Autodesk Inventor part; units mm, degrees
ref_plane "YZ Plane" through (0, 0, 0) normal (1, 0, 0) x (0, 1, 0)
ref_plane "XZ Plane" through (0, 0, 0) normal (0, 1, 0) x (-1, 0, 0)
ref_plane "XY Plane" through (0, 0, 0) normal (0, 0, 1) x (1, 0, 0)
sketch "Sketch1" plane through (0, 0, 0) normal (0, 1, 0) x (-1, 0, 0)
  line L0 (33.5, -13.5) -> (-33.5, -13.5)
  line L1 (-33.5, -13.5) -> (-33.5, 13.5)
  line L2 (-33.5, 13.5) -> (33.5, 13.5)
  line L3 (33.5, 13.5) -> (33.5, -13.5)
  line L4 (0, 0) -> (86.7229, 0) construction
  line L5 (0, 0) -> (0, 45.1017) construction
  dimension "d0" = 27
  dimension "d1" = 67
extrude "Extrusion1" add sketch "Sketch1" along normal blind 3
sketch "Sketch2" plane through (0, 3, 0) normal (0, 1, 0) x (1, 0, 0)
  line L0 (33.5, 13.5) -> (-33.5, 13.5)
  line L1 (33.5, -13.5) -> (33.5, 13.5)
  line L2 (0, 0) -> (26.8835, 0) construction
  line L3 (0, 0) -> (0, 11.9949) construction
  circle A0 centre (30, 9) radius 2.15
  circle A1 centre (-30, 9) radius 2.15
  circle A2 centre (30, -9) radius 2.15
  circle A3 centre (-30, -9) radius 2.15
  dimension "d4" = 4.3
  dimension "d5" = 3.5
  dimension "d6" = 4.5
extrude "Extrusion2" cut sketch "Sketch2" against normal through all
fillet "Fillet1" radius 2 4 edges at (-33.5, 1.5, 13.5) (-33.5, 1.5, -13.5) (33.5, 1.5, -13.5) (33.5, 1.5, 13.5)
sketch "Sketch3" plane through (0, 3, 0) normal (0, 1, 0) x (1, 0, 0)
  line L0 (33.5, -11.5) -> (33.5, 11.5)
  line L1 (23.5, 6) -> (33.5, 6)
  line L2 (33.5, 6) -> (33.5, -6)
  line L3 (33.5, -6) -> (23.5, -6)
  line L4 (23.5, -6) -> (23.5, 6)
  line L5 (0, 0) -> (50.7888, 0) construction
  line L6 (23.5, 10) -> (-21.5, 10)
  line L7 (-21.5, 10) -> (-21.5, -10)
  line L8 (-21.5, -10) -> (23.5, -10)
  line L9 (23.5, -10) -> (23.5, 10)
  dimension "d10" = 10
  dimension "d11" = 12
  dimension "d12" = 20
  dimension "d13" = 45
extrude "Extrusion3" add sketch "Sketch3" along normal blind 9
sketch "Sketch4" plane through (0, 3, 0) normal (0, 1, 0) x (1, 0, 0)
  line L0 (-33.5, 11.5) -> (-33.5, -11.5)
  line L1 (-33.5, 4) -> (-27.5, 4)
  line L2 (-27.5, 4) -> (-27.5, -4)
  line L3 (-27.5, -4) -> (-33.5, -4)
  line L4 (-33.5, -4) -> (-33.5, 4)
  line L5 (0, 0) -> (-50.5157, 0) construction
  dimension "d16" = 6
  dimension "d17" = 8
extrude "Extrusion4" add sketch "Sketch4" along normal blind 3
fillet "Fillet2" radius 2 2 edges at (-30.5, 6, 4) (-30.5, 6, -4)
properties part number "Board"
Model file for the job. Use its own axes, mm. A direction names the side the tool comes from. Round coordinates to 2 decimals unless told otherwise and drop trailing zeros. Loops run counter-clockwise (first coordinate to the right, second up) from the corner with the lowest first, then second, coordinate; pieces in that order, holes last. Notation, with made-up numbers: M 82.5,24 L 139.5,24 A22 ccw 139.5,60 Z; hole C 45.5,86 d11. An arc over 180 degrees is marked long. Put each result on its own line as item: value. Start each with the question number.
Item 1: Mould opens along Z. For faces 1 (the face through (-27.95, 1.52, -9.65)), 2 (the face through (1, 7, 10)), 3 (the face through (-21.5, 7, 0)) say: released by +Z, released by -Z, zero draft, split by the parting line, or undercut.
Item 2: 3-axis set-ups, long thin cutter, end or side, ignore diameter. For faces 4 (the face through (-30.46, 5.4, -3.43)), 5 (the face through (1, 7, -10)), 6 (the face through (29, 7, 6)), 7 (the face through (28, 7, -6)): which of +Z, -Z, +X, -X, +Y, -Y reach the whole face in a straight line?
Item 3: Drill centre lines: line 1 along X through (y, z) = (2.1, 9); line 2 along Z through (x, y) = (30, 1.35); line 3 along X through (y, z) = (5.75, 0). Where is each one in solid material? Low to high.
Item 4: Drop flat-ended pins along their axis: P1, Ø2, axis at x = -4, y = 8.5, coming from the +Z side; P2, Ø4.5, axis at x = 9, y = 6, coming from the -Z side; P3, Ø2, axis at x = -31.5, z = 0, coming from the +Y side. Give the stop position or say it passes through.
Item 5: Cut at A-A (x = 30). List the corners of the cut face in (y, z).
Item 6: Cut at B-B (y = 1). List the corners of the cut face in (x, z), then the cut area to 3 significant figures.
Item 7: Cut at D-D (x = -5.5). List the corners of the cut face in (y, z).
Item 8: Cut at C-C (z = 9). List the corners of the cut face in (x, y).
Answer block:
1. face 1: undercut
1. face 2: released by +Z
1. face 3: zero draft
2. face 4: -Z, -X, +Y
2. face 5: -Z, +X, -X, +Y
2. face 6: +Z, +X, +Y
2. face 7: -Z, +X, +Y
3. line 1: -33.5 to -32.15, -27.85 to 27.85, 32.15 to 33.5
3. line 2: -13.5 to -11.15, -6.85 to 6.85, 11.15 to 13.5
3. line 3: -33.5 to -27.5, -21.5 to 33.5
4. P1: z = 10
4. P2: z = -10
4. P3: y = 6
5. outline: M 0,-13.5 L 3,-13.5 L 3,-11.15 L 0,-11.15 Z; M 0,-6.85 L 3,-6.85 L 3,-6 L 12,-6 L 12,6 L 3,6 L 3,6.85 L 0,6.85 Z; M 0,11.15 L 3,11.15 L 3,13.5 L 0,13.5 Z
6. outline: M -33.5,-11.5 A2 ccw -31.5,-13.5 L 31.5,-13.5 A2 ccw 33.5,-11.5 L 33.5,11.5 A2 ccw 31.5,13.5 L -31.5,13.5 A2 ccw -33.5,11.5 Z; hole C -30,-9 d4.3; hole C -30,9 d4.3; hole C 30,-9 d4.3; hole C 30,9 d4.3
6. area: 1,750 mm2
7. outline: M 0,-13.5 L 3,-13.5 L 3,-10 L 12,-10 L 12,10 L 3,10 L 3,13.5 L 0,13.5 Z
8. outline: M -33.5,0 L -32.15,0 L -32.15,3 L -33.5,3 Z; M -27.85,0 L 27.85,0 L 27.85,3 L 23.5,3 L 23.5,12 L -21.5,12 L -21.5,3 L -27.85,3 Z; M 32.15,0 L 33.5,0 L 33.5,3 L 32.15,3 Z
